```python
from build123d import *

# Parameters (mm, degrees)
BOSS_EXTRUDE1_DEPTH = 47
SKETCH2_R           = 1.5
CUT_EXTRUDE1_DEPTH  = 4
SKETCH3_R           = 8
CUT_EXTRUDE2_DEPTH  = 9.560785614
SKETCH4_R           = 1.47
CUT_EXTRUDE3_DEPTH  = 9.560785614


with BuildPart() as part:
    # Sketch1 → Boss-Extrude1 (new body)
    with BuildSketch(Plane(origin=(0, 0, 0), x_dir=(1, 0, 0), z_dir=(0, 1, 0))):
        with BuildLine():
            Line((-2.32059976, 10.913457617), (11.001200978, 10.913457617))
            ThreePointArc((11.001200978, 10.913457617), (14.215139026, 9.743679833), (15.925239743, 6.781698506))
            Line((15.925239743, 6.781698506), (20.843268829, -21.10983044))
            Line((20.843268829, -21.10983044), (17.88884557, -21.630774973))
            Line((17.88884557, -21.630774973), (13.407940849, 3.781698506))
            ThreePointArc((13.407940849, 3.781698506), (11.697840132, 6.743679833), (8.483902084, 7.913457617))
            Line((8.483902084, 7.913457617), (-2.32059976, 7.913457617))
            Line((-2.32059976, 7.913457617), (-2.32059976, 10.913457617))
        make_face()
    extrude(amount=BOSS_EXTRUDE1_DEPTH)

    # Sketch2 → Cut-Extrude1 (cut, through all)
    with BuildSketch(Plane.XY.offset(-7.913457617)):
        with Locations((2.67940024, 30)):
            Circle(SKETCH2_R)
        with Locations((2.67940024, 17)):
            Circle(SKETCH2_R)
    extrude(amount=-CUT_EXTRUDE1_DEPTH, mode=Mode.SUBTRACT)

    # Sketch3 → Cut-Extrude2 (cut, through all)
    with BuildSketch(Plane(origin=(13.650350495, 0, -2.406925088), x_dir=(0.173648178, 0, 0.984807753), z_dir=(-0.984807753, 0, 0.173648178))):
        with BuildLine():
            Line((24.408520331, 47), (13.408520331, 47))
            ThreePointArc((13.408520331, 47), (21.186694924, 43.778174593), (24.408520331, 36))
            Line((24.408520331, 36), (24.408520331, 47))
        make_face()
        with BuildLine():
            Line((24.408520331, 0), (24.408520331, 11))
            ThreePointArc((24.408520331, 11), (21.186694924, 3.221825407), (13.408520331, 0))
            Line((13.408520331, 0), (24.408520331, 0))
        make_face()
        with Locations((13.408520331, 11)):
            Circle(SKETCH3_R)
        with Locations((13.408520331, 36)):
            Circle(SKETCH3_R)
        with BuildLine():
            Line((24.408520331, 11), (24.408520331, 36))
            ThreePointArc((24.408520331, 36), (22.930853605, 30.493170692), (18.894853235, 26.465842918))
            ThreePointArc((18.894853235, 26.465842918), (17.17968635, 23.5), (18.894853235, 20.534157082))
            ThreePointArc((18.894853235, 20.534157082), (22.930853605, 16.506829308), (24.408520331, 11))
        make_face()
    extrude(amount=-CUT_EXTRUDE2_DEPTH, mode=Mode.SUBTRACT)

    # Sketch4 → Cut-Extrude3 (cut, through all)
    with BuildSketch(Plane(origin=(13.650350495, 0, -2.406925088), x_dir=(0.173648178, 0, 0.984807753), z_dir=(-0.984807753, 0, 0.173648178))):
        with Locations((3.604018487, 27.463505193)):
            Circle(SKETCH4_R)
        with Locations((3.604018487, 19.536494807)):
            Circle(SKETCH4_R)
    extrude(amount=-CUT_EXTRUDE3_DEPTH, mode=Mode.SUBTRACT)


solid = part.part
```
For this review, take the finished solid that the model builds, in its own axes (mm). A direction names the side the tool comes from. Coordinates: 2 decimals unless noted, no trailing zeros. Loops run counter-clockwise (first coordinate to the right, second up) from the corner with the lowest first, then second, coordinate; pieces in that order, holes last. Notation, with made-up numbers: (-27.75, -13.75) -> (-23.75, -13.75) arc R15 ccw to (-23.75, 1.25) -> close; hole circle Ø2 at (4.5, 55.25). An arc over 180 degrees is marked (long way). Return JSON: item names as keys, results as strings. Group by question number.
(1) Mouldability with a two-part tool opening along Z and no side actions: class faces 3 (the flat face through (13, 47, -6)), 4 (the cylindrical face through (15.68, 18.1, 0.57)), 5 (the flat face through (4, 23, -10.913)) as pulls with the +Z half, pulls with the -Z half, needs draft (parallel to the pull), parting line crosses it, or undercut.
(2) Consider section A-A, the plane x = 2. Give the boundary of the cut face in (y, z).
(3) Consider section D-D, the plane x = 5.5. Give the boundary of the cut face in (y, z), plus the area to 3 significant figures.
(4) Consider section C-C, the plane z = 7. Count the separate pieces of the cut face and the enclosed holes in it, plus the area to 3 significant figures.
(5) Consider section B-B, the plane y = 30. Give the boundary of the cut face in (x, z).
(6) For pin 1 Ø3.5 at (x, y) = (2.68, 30) entering from +Z; pin 2 Ø2 at (y, z) = (36.5, -1.5) entering from -X; pin 3 Ø3 at (y, z) = (5, 14) entering from +X; pin 4 Ø4 at (x, z) = (1, -4) entering from +Y, all flat-tipped, find the tip position at first contact; note any pin that passes through.
(7) Tool access review of faces 1 (the cylindrical face through (1.57, 18.01, -9.39)), 2 (the flat face through (3, 23, -7.913)): name each direction out of +Z, -Z, +X, -X, +Y, -Y from which nothing blocks a thin tool from reaching the whole face with its end or side.
(8) To check wall thickness, follow L1, parallel to Y at x = 17.75, z = 13.5; L2, parallel to Y at x = 18, z = 12; L3, parallel to Z at x = 5, y = 10.5. State the ranges of each line that lie inside material, in increasing order.
Results below:
{
 "1": {"face 3": "needs draft", "face 4": "undercut", "face 5": "pulls with the -Z half"},
 "2": {"outline": "(0, -10.91) -> (15.66, -10.91) -> (15.66, -7.91) -> (0, -7.91) -> close; (18.34, -10.91) -> (28.66, -10.91) -> (28.66, -7.91) -> (18.34, -7.91) -> close; (31.34, -10.91) -> (47, -10.91) -> (47, -7.91) -> (31.34, -7.91) -> close"},
 "3": {"outline": "(0, -10.91) -> (47, -10.91) -> (47, -7.91) -> (0, -7.91) -> close", "area": "141 mm2"},
 "4": {"separate pieces": "3", "enclosed holes": "0", "area": "56.1 mm2"},
 "5": {"outline": "(-2.32, -10.91) -> (1.18, -10.91) -> (1.18, -7.91) -> (-2.32, -7.91) -> close; (4.18, -10.91) -> (11, -10.91) arc R5 ccw to (15.93, -6.78) -> (18.01, 5.07) -> (15.06, 5.59) -> (13.41, -3.78) arc R5 cw to (8.48, -7.91) -> (4.18, -7.91) -> close; (16.9, 16.01) -> (19.85, 15.49) -> (20.53, 19.36) -> (17.58, 19.88) -> close"},
 "6": {"pin 1": "stops at z = -7.91", "pin 2": "stops at x = 13.63", "pin 3": "stops at x = 19.85", "pin 4": "passes through"},
 "7": {"face 1": "+Z, -Z", "face 2": "+Z, -X, +Y, -Y"},
 "8": {"L1": "y = 0.41 to 3.57, 18.43 to 28.57, 43.43 to 46.59", "L2": "y = 0.11 to 3.15, 18.85 to 28.15, 43.85 to 46.89", "L3": "z = -10.91 to -7.91"}
}
